Study the drawing (mm; zero at the part's minimum x, y, z) and answer. Coordinates: 2 decimals unless noted, no trailing zeros. Loops run counter-clockwise (first coordinate to the right, second up) from the corner with the lowest first, then second, coordinate; pieces in that order, holes last. Notation, with made-up numbers: (37.5, 36) - (67.5, 36) arc R27 cw to (67.5, 57) - close; hole circle Ø2 at (36, 52.25). An arc over 180 degrees is marked (long way). Write each question's results on one line, items separated by ' | '. Start each with the question number.
(1) Given pin 1 Ø1 at (y, z) = (2, 2) entering from +X (1 decimal); pin 2 Ø1 at (x, y) = (27, 2) entering from -Z; pin 3 Ø0.5 at (y, z) = (1, 2) entering from -X, each flat-ended and moving along its own axis, determine where each tip first touches the part or whether it passes through.
(2) Find section C-C on z = 3. Determine the outline of the cut face in (x, y) (1 decimal).
(3) Find section A-A on y = 1.65. Determine the outline of the cut face in (x, z).
(4) Consider line 1 (X direction, y = 2.85, z = 2.5) (1 decimal); line 2 (Z direction, x = 2, y = 1.9); line 3 (Z direction, x = 3.5, y = 0.55) (1 decimal). Determine where each line is inside the solid, lowest interval first. Write a range as from..to.
(5) Find section B-B on x = 25.25. Determine the outline of the cut face in (y, z) (1 decimal).
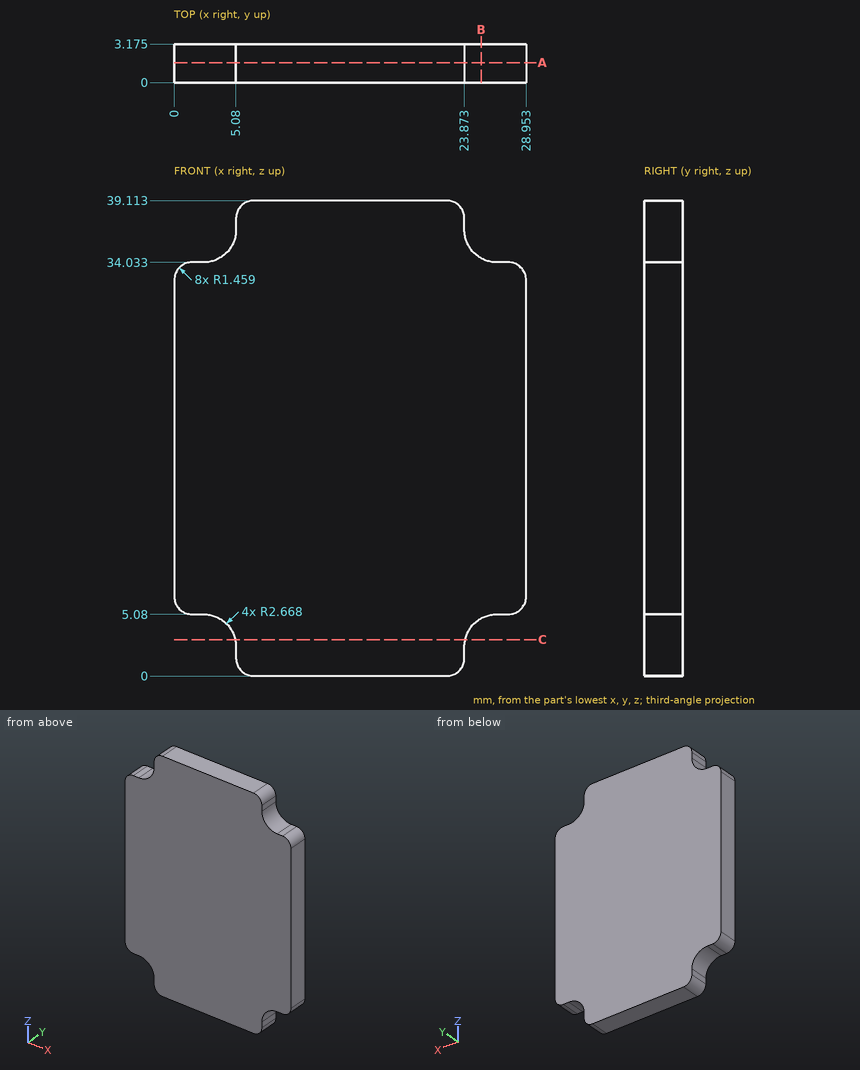
Values:
1) pin 1: stops at x = 23.9 | pin 2: stops at z = 5.08 | pin 3: stops at x = 5.08
2) outline: (5, 0) - (23.9, 0) - (23.9, 3.2) - (5, 3.2) - close
3) outline: (0, 6.54) arc R1.46 ccw to (1.46, 5.08) - (2.41, 5.08) arc R2.67 cw to (5.08, 2.41) - (5.08, 1.46) arc R1.46 ccw to (6.54, 0) - (22.41, 0) arc R1.46 ccw to (23.87, 1.46) - (23.87, 2.41) arc R2.67 cw to (26.54, 5.08) - (27.49, 5.08) arc R1.46 ccw to (28.95, 6.54) - (28.95, 32.57) arc R1.46 ccw to (27.49, 34.03) - (26.54, 34.03) arc R2.67 cw to (23.87, 36.7) - (23.87, 37.65) arc R1.46 ccw to (22.41, 39.11) - (6.54, 39.11) arc R1.46 ccw to (5.08, 37.65) - (5.08, 36.7) arc R2.67 cw to (2.41, 34.03) - (1.46, 34.03) arc R1.46 ccw to (0, 32.57) - close
4) line 1: x = 5.1..23.9 | line 2: z = 5.08..34.03 | line 3: z = 4.8..34.3
5) outline: (0, 4.7) - (3.2, 4.7) - (3.2, 34.4) - (0, 34.4) - close
